The listing builds one solid part. Answer for the finished solid, in the listing's coordinates (mm). Face numbers are marked on the shaded views. A direction names the side the tool comes from. Give positions to 0.01 mm unless a question says otherwise; leave off trailing zeros. Write each loop counter-clockwise with the first axis right and the second up, starting at its lowest first coordinate (ties: lowest second). Pieces come first, ordered by that corner, then holes. Notation, with made-up numbers: (-11.5, -23.5) - (29.5, -23.5) arc R17 ccw to (29.5, -13.5) - close; hole circle Ø7 at (46.5, 33.25). An arc over 180 degrees is marked (long way). One line per question, with ' | ' between items. Start each with the question number.
1. A cutting plane is placed at D-D (x = 44.45). Determine the outline of the cut face in (y, z).
2. A cutting plane is placed at A-A (z = -1). State how many separate pieces and enclosed holes the cut face has, then the cut area to 3 significant figures.
3. Given P1, Ø1.5, axis at x = 6.5, z = -2, coming from the +Y side; P2, Ø1.5, axis at x = 37, z = -5.5, coming from the -Y side; P3, Ø5, axis at x = -6.35, y = 0, coming from the -Z side, each flat-ended and moving along its own axis, determine where each tip first touches the part or whether it passes through.
4. Find the intervals of material crossed by L1, parallel to Z at x = 37.5, y = -3.5; L2, parallel to Z at x = -4, y = -5; L3, parallel to Z at x = -8.5, y = 2.5, in increasing order. Write a range as from..to.
5. For the marked faces 1, 2 and 3, determine the directions among +Z, -Z, +X, -X, +Y, -Y from which every point of the face is accessible in a straight line to the end or side of a thin tool.
6. A cutting plane is placed at C-C (x = 9.5). Determine the outline of the cut face in (y, z), then the cut area to 3 significant figures.
```python
from build123d import *

# Parameters (mm, degrees)
SKETCH4_R                  = 3.9624
SKETCH4_R_2                = 2.0066
BOSS_EXTRUDE1_DEPTH        = 3.96875
BOSS_EXTRUDE1_2_DEPTH      = 3.96875
SKETCH5_R                  = 1.9812
BOSS_EXTRUDE2_DEPTH        = 1.524
LPATTERN1_COUNT            = 2
LPATTERN1_PITCH            = 12.7
SKETCH7_R                  = 1.9812
BOSS_EXTRUDE3_DEPTH        = 1.524
SKETCH8_R                  = 1.9812
BOSS_EXTRUDE4_DEPTH        = 8.2042
BOSS_EXTRUDE4_DEPTH_BACK   = 8.2042
BOSS_EXTRUDE4_2_DEPTH      = 8.2042
BOSS_EXTRUDE4_2_DEPTH_BACK = 8.2042
LPATTERN2_COUNT            = 2
LPATTERN2_PITCH            = 25.4


with BuildPart() as part:
    # Sketch4 → Boss-Extrude1 (new body, symmetric)
    with BuildSketch(Plane.XY):
        with Locations((-6.35, 0)):
            Circle(SKETCH4_R)
        with Locations((-6.35, 0)):
            Circle(SKETCH4_R_2, mode=Mode.SUBTRACT)
    extrude(amount=BOSS_EXTRUDE1_DEPTH, both=True)


with BuildPart() as body_2:
    # Sketch4 → Boss-Extrude1 2 (new body, symmetric)
    with BuildSketch(Plane.XY):
        with Locations((6.35, 0)):
            Circle(SKETCH4_R)
        with Locations((6.35, 0)):
            Circle(SKETCH4_R_2, mode=Mode.SUBTRACT)
    extrude(amount=BOSS_EXTRUDE1_2_DEPTH, both=True)


with BuildPart() as body_3:
    # Sketch5 → Boss-Extrude2 (new body)
    with BuildSketch(Plane.XY.offset(3.96875)):
        with BuildLine():
            ThreePointArc((-4.787931893, 5.589740462), (-12.1539, 0), (-4.787931893, -5.589740462))
            ThreePointArc((-4.787931893, -5.589740462), (0, -4.933315), (4.787931893, -5.589740462))
            ThreePointArc((4.787931893, -5.589740462), (12.1539, 0), (4.787931893, 5.589740462))
            ThreePointArc((4.787931893, 5.589740462), (0, 4.933315), (-4.787931893, 5.589740462))
        make_face()
        with Locations((-6.35, 0)):
            Circle(SKETCH5_R, mode=Mode.SUBTRACT)
        with Locations((6.35, 0)):
            Circle(SKETCH5_R, mode=Mode.SUBTRACT)
    extrude(amount=BOSS_EXTRUDE2_DEPTH)


with BuildPart() as lpattern1_1:
    # LPattern1: pattern copy
    add(body_2.part.moved(Location(Vector(1, 0, 0) * (1 * LPATTERN1_PITCH))))


with BuildPart() as body_5:
    # Sketch7 → Boss-Extrude3 (new body)
    with BuildSketch(Plane.XY.offset(-5.54355)):
        with BuildLine():
            ThreePointArc((7.766432158, 4.907095024), (1.242568, 0), (7.766432158, -4.907095024))
            ThreePointArc((7.766432158, -4.907095024), (12.7, -4.209302295), (17.633567842, -4.907095024))
            ThreePointArc((17.633567842, -4.907095024), (24.157432, 0), (17.633567842, 4.907095024))
            ThreePointArc((17.633567842, 4.907095024), (12.7, 4.209302295), (7.766432158, 4.907095024))
        make_face()
        with Locations((6.35, 0)):
            Circle(SKETCH7_R, mode=Mode.SUBTRACT)
        with Locations((19.05, 0)):
            Circle(SKETCH7_R, mode=Mode.SUBTRACT)
    extrude(amount=-BOSS_EXTRUDE3_DEPTH)


with BuildPart() as body_6:
    # Mirror1: mirrored copy
    add(body_3.part.mirror(Plane.XY))


with BuildPart() as body_7:
    # Mirror1 2: mirrored copy
    add(body_5.part.mirror(Plane.XY))


with BuildPart() as body_8:
    # Sketch8 → Boss-Extrude4 (new body, two sides)
    with BuildSketch(Plane.XY) as boss_extrude4_sk:
        with Locations((6.35, 0)):
            Circle(SKETCH8_R)
    extrude(amount=BOSS_EXTRUDE4_DEPTH)
    extrude(boss_extrude4_sk.sketch, amount=-BOSS_EXTRUDE4_DEPTH_BACK)


with BuildPart() as body_9:
    # Sketch8 → Boss-Extrude4 2 (new body, two sides)
    with BuildSketch(Plane.XY) as boss_extrude4_2_sk:
        with Locations((19.05, 0)):
            Circle(SKETCH8_R)
    extrude(amount=BOSS_EXTRUDE4_2_DEPTH)
    extrude(boss_extrude4_2_sk.sketch, amount=-BOSS_EXTRUDE4_2_DEPTH_BACK)


with BuildPart() as lpattern2_1:
    # LPattern2: pattern copy
    add(body_9.part.moved(Location(Vector(1, 0, 0) * (1 * LPATTERN2_PITCH))))


with BuildPart() as lpattern2_2:
    # LPattern2: pattern copy
    add(body_8.part.moved(Location(Vector(1, 0, 0) * (1 * LPATTERN2_PITCH))))


with BuildPart() as lpattern2_3:
    # LPattern2: pattern copy
    add(body_7.part.moved(Location(Vector(1, 0, 0) * (1 * LPATTERN2_PITCH))))


with BuildPart() as lpattern2_4:
    # LPattern2: pattern copy
    add(body_6.part.moved(Location(Vector(1, 0, 0) * (1 * LPATTERN2_PITCH))))


with BuildPart() as lpattern2_5:
    # LPattern2: pattern copy
    add(body_5.part.moved(Location(Vector(1, 0, 0) * (1 * LPATTERN2_PITCH))))


with BuildPart() as lpattern2_6:
    # LPattern2: pattern copy
    add(lpattern1_1.part.moved(Location(Vector(1, 0, 0) * (1 * LPATTERN2_PITCH))))


with BuildPart() as lpattern2_7:
    # LPattern2: pattern copy
    add(body_3.part.moved(Location(Vector(1, 0, 0) * (1 * LPATTERN2_PITCH))))


with BuildPart() as lpattern2_8:
    # LPattern2: pattern copy
    add(body_2.part.moved(Location(Vector(1, 0, 0) * (1 * LPATTERN2_PITCH))))


with BuildPart() as lpattern2_9:
    # LPattern2: pattern copy
    add(part.part.moved(Location(Vector(1, 0, 0) * (1 * LPATTERN2_PITCH))))


with BuildPart() as body_2_1:
    add(body_2.part)

    # Combine1: union body 3, LPattern1_1, body 5, body 6, body 7, body 8, body 9, LPattern2_1, LPattern2_2, LPattern2_3, LPattern2_4, LPattern2_5, LPattern2_7, LPattern2_8, LPattern2_9, part
    add(body_3.part)
    add(lpattern1_1.part)
    add(body_5.part)
    add(body_6.part)
    add(body_7.part)
    add(body_8.part)
    add(body_9.part)
    add(lpattern2_1.part)
    add(lpattern2_2.part)
    add(lpattern2_3.part)
    add(lpattern2_4.part)
    add(lpattern2_5.part)
    add(lpattern2_7.part)
    add(lpattern2_8.part)
    add(lpattern2_9.part)
    add(part.part)


solid = body_2_1.part
```
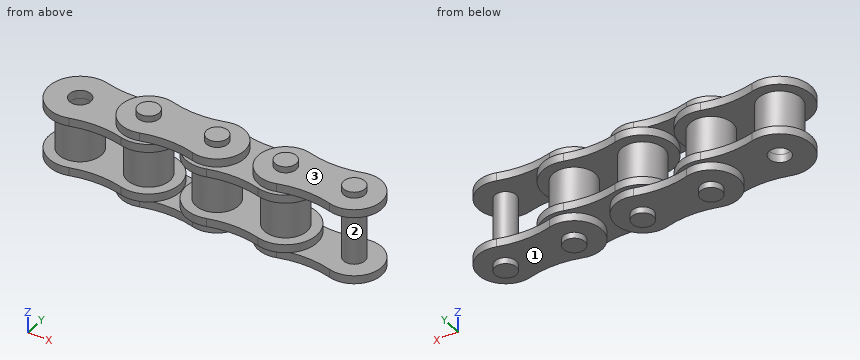
Determined:
1) outline: (-5.11, -7.07) - (-1.98, -7.07) - (-1.98, -8.2) - (1.98, -8.2) - (1.98, -7.07) - (5.11, -7.07) - (5.11, -5.54) - (1.98, -5.54) - (1.98, 5.54) - (5.11, 5.54) - (5.11, 7.07) - (1.98, 7.07) - (1.98, 8.2) - (-1.98, 8.2) - (-1.98, 7.07) - (-5.11, 7.07) - (-5.11, 5.54) - (-1.98, 5.54) - (-1.98, -5.54) - (-5.11, -5.54) - close
2) separate pieces: 8 | enclosed holes: 4 | area: 196 mm2
3) P1: y = 3.96 | P2: y = -4.31 | P3: z = -5.49
4) L1: -7.07..-5.54, 5.54..7.07 | L2: -5.49..-3.97, 3.97..5.49 | L3: -5.49..5.49
5) face 1: -Z | face 2: none | face 3: +Z
6) outline: (-4.87, -5.49) - (4.87, -5.49) - (4.87, -3.97) - (2.4, -3.97) - (2.4, 3.97) - (4.87, 3.97) - (4.87, 5.49) - (-4.87, 5.49) - (-4.87, 3.97) - (-2.4, 3.97) - (-2.4, -3.97) - (-4.87, -3.97) - close; (-4.5, -7.07) - (4.5, -7.07) - (4.5, -5.54) - (-4.5, -5.54) - close; (-4.5, 5.54) - (4.5, 5.54) - (4.5, 7.07) - (-4.5, 7.07) - close | area: 95.3 mm2
